CAD build for the part. Positions are in the model's coordinates, mm. Face numbers are marked on the shaded views. A direction names the side the tool comes from. Give positions to 0.01 mm unless a question says otherwise; leave off trailing zeros. Order: outer loops, then holes, each group sorted by start corner. A loop starts at its lowest first (then second) coordinate and runs counter-clockwise, first axis right, second up.
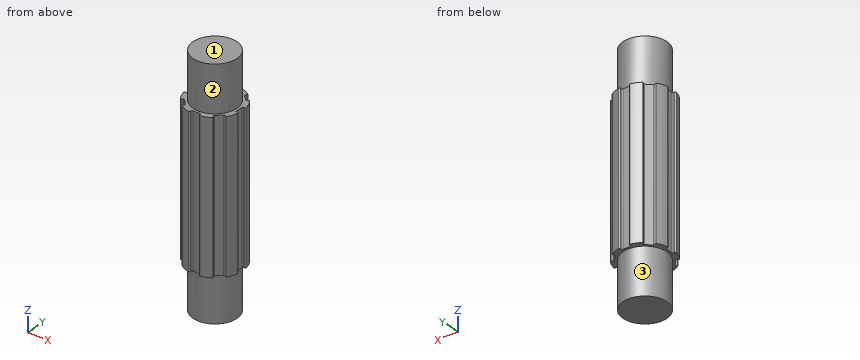
from build123d import *

# Parameters (mm, degrees)
SKETCH1_R                = 6
BOSS_EXTRUDE1_DEPTH      = 26.095
SKETCH2_OUTSIDE_W        = 24.976
SKETCH2_OUTSIDE_H        = 24.976
SKETCH2_OUTSIDE_R        = 4.75
CUT_EXTRUDE1_DEPTH       = 10
SKETCH3_W                = 2
SKETCH3_H                = 2
CUT_EXTRUDE2_DEPTH       = 28.439916636
FILLET1_R                = 0.2
CIRPATTERN1_COUNT        = 8
FILLET1_OF_CIRPATTERN1_R = 0.2


with BuildPart() as part:
    # Sketch1 → Boss-Extrude1 (new, symmetric)
    with BuildSketch(Plane.XY):
        Circle(SKETCH1_R)
    extrude(amount=BOSS_EXTRUDE1_DEPTH, both=True)

    # Sketch2 outside → Cut-Extrude1 (cut)
    with BuildSketch(Plane.XY.offset(26.095)):
        Rectangle(SKETCH2_OUTSIDE_W, SKETCH2_OUTSIDE_H)
        Circle(SKETCH2_OUTSIDE_R, mode=Mode.SUBTRACT)
    cut_extrude1 = extrude(amount=-CUT_EXTRUDE1_DEPTH, mode=Mode.SUBTRACT)

    # Mirror1: Cut-Extrude1 across plane
    add(cut_extrude1.mirror(Plane.XY), mode=Mode.SUBTRACT)

    # Sketch3 → Cut-Extrude2 (cut, symmetric)
    with BuildSketch(Plane.XY):
        with Locations((0, 6.25)):
            Rectangle(SKETCH3_W, SKETCH3_H)
    cut_extrude2 = extrude(amount=CUT_EXTRUDE2_DEPTH, both=True, mode=Mode.SUBTRACT)

    # Fillet1
    fillet1_edges = [part.edges().sort_by_distance(p)[0] for p in [
        (1, 5.916079783, 0),
        (1, 5.25, 0),
        (-1, 5.916079783, 0),
        (-1, 5.25, 0),
    ]]
    fillet(fillet1_edges, radius=FILLET1_R)

    # CirPattern1: Cut-Extrude2 ×8 about axis
    cirpattern1_axis = Axis((0, 0, 0), (0, 0, 1))
    for i in range(1, CIRPATTERN1_COUNT):
        add(cut_extrude2.rotate(cirpattern1_axis, i * 360 / CIRPATTERN1_COUNT), mode=Mode.SUBTRACT)

    # Fillet1 of CirPattern1
    fillet1_of_cirpattern1_edges = [part.edges().sort_by_distance(p)[0] for p in [
        (-3.476193351, 4.890406914, 0),
        (-3.00520382, 4.419417382, 0),
        (-4.890406914, 3.476193351, 0),
        (-4.419417382, 3.00520382, 0),
        (-5.916079783, 1, 0),
        (-5.25, 1, 0),
        (-5.916079783, -1, 0),
        (-5.25, -1, 0),
        (-4.890406914, -3.476193351, 0),
        (-4.419417382, -3.00520382, 0),
        (-3.476193351, -4.890406914, 0),
        (-3.00520382, -4.419417382, 0),
        (-1, -5.916079783, 0),
        (-1, -5.25, 0),
        (1, -5.916079783, 0),
        (1, -5.25, 0),
        (3.476193351, -4.890406914, 0),
        (3.00520382, -4.419417382, 0),
        (4.890406914, -3.476193351, 0),
        (4.419417382, -3.00520382, 0),
        (5.916079783, -1, 0),
        (5.25, -1, 0),
        (5.916079783, 1, 0),
        (5.25, 1, 0),
        (4.890406914, 3.476193351, 0),
        (4.419417382, 3.00520382, 0),
        (3.476193351, 4.890406914, 0),
        (3.00520382, 4.419417382, 0),
    ]]
    fillet(fillet1_of_cirpattern1_edges, radius=FILLET1_OF_CIRPATTERN1_R)


solid = part.part
1. Saw through at A-A on x = 0. Give the cut face in (y, z) (3 decimals).
2. 3-axis set-ups, long thin cutter, end or side, ignore diameter. For the marked faces 1, 2 and 3: which of +Z, -Z, +X, -X, +Y, -Y reach the whole face in a straight line?
3. Wall check: line 1 (Z direction, x = 3, y = -4.25) (3 decimals); line 2 (X direction, y = -0.5, z = -2.5); line 3 (X direction, y = -0.25, z = -22). Give the ranges that are in metal, low to high.
4. Saw through at C-C on z = -18. Give the cut face in (x, y).
5. Pin check, flat tips, straight feed: P1, Ø1, axis at x = 4, y = -4, coming from the -Z side (3 decimals); P2, Ø1.3, axis at x = 0, z = 5.5, coming from the +Y side; P3, Ø0.5, axis at y = 0, z = 1.5, coming from the +X side. Stop position of each tip, or through.
Reported:
1. outline: (-5.25, -16.095) - (-4.75, -16.095) - (-4.75, -26.095) - (4.75, -26.095) - (4.75, -16.095) - (5.25, -16.095) - (5.25, 16.095) - (4.75, 16.095) - (4.75, 26.095) - (-4.75, 26.095) - (-4.75, 16.095) - (-5.25, 16.095) - close
2. face 1: +Z, +X, -X, +Y, -Y
2. face 2: +Z
2. face 3: -Z
3. line 1: z = -16.095 to 16.095
3. line 2: x = -5.25 to 5.25
3. line 3: x = -4.74 to 4.74
4. outline: circle Ø9.5 at (0, 0)
5. P1: stops at z = -16.095
5. P2: stops at y = 5.25
5. P3: stops at x = 5.25
